```python
from build123d import *

# Parameters (mm, degrees)
ESQUISSE1_W             = 32.4
ESQUISSE1_H             = 21
BOSS_EXTRU_1_DEPTH      = 4
ESQUISSE2_W             = 4.7
ESQUISSE2_H             = 9.85
BOSS_EXTRU_2_DEPTH      = 12.3
ENL_V_MAT_EXTRU_1_REACH = 33.528
ESQUISSE3_R             = 0.95
CHANFREIN1_SIZE         = 1.915
CHANFREIN1_SIZE2        = 1.6
ESQUISSE4_R             = 1
ENL_V_MAT_EXTRU_2_DEPTH = 10
CONG_1_R                = 4.5
ESQUISSE5_R             = 1.5
ENL_V_MAT_EXTRU_3_DEPTH = 30.657924742
CHANFREIN2_SIZE         = 2.915
CHANFREIN2_SIZE2        = 2.24


with BuildPart() as part:
    # Esquisse1 → Boss.-Extru.1 (new body)
    with BuildSketch(Plane(origin=(0, 0, 0), x_dir=(1, 0, 0), z_dir=(0, 1, 0))):
        with Locations((0.75, -10.5)):
            Rectangle(ESQUISSE1_W, ESQUISSE1_H)
    extrude(amount=BOSS_EXTRU_1_DEPTH)

    # Esquisse2 → Boss.-Extru.2 (add)
    with BuildSketch(Plane(origin=(0, 4, 0), x_dir=(1, 0, 0), z_dir=(0, 1, 0))):
        Polygon((-15.45, 0), (-10.75, 0), (-10.75, -16.3), (16.95, -16.3), (16.95, -21), (-15.45, -21), align=None)
        with Locations((14.6, -4.925)):
            Rectangle(ESQUISSE2_W, ESQUISSE2_H)
    extrude(amount=BOSS_EXTRU_2_DEPTH)

    # Esquisse3 → Enlèv. mat.-Extru.1 (cut, up to next)
    with BuildSketch(Plane.XY.offset(21), mode=Mode.PRIVATE) as enl_v_mat_extru_1_sk1:
        with Locations((6.268372061, 10)):
            Circle(ESQUISSE3_R)
    enl_v_mat_extru_1_tool1 = extrude(enl_v_mat_extru_1_sk1.sketch, amount=-ENL_V_MAT_EXTRU_1_REACH, mode=Mode.PRIVATE) & part.part
    add(enl_v_mat_extru_1_tool1.solids().sort_by_distance((6.268372, 10, 21))[0], mode=Mode.SUBTRACT)

    # Chanfrein1
    chanfrein1_edges = [part.edges().sort_by_distance(p)[0] for p in [
        (5.318372061, 10, 16.3),
    ]]
    chanfrein1_side = [part.faces().sort_by_distance(p)[0] for p in [
        (3.073412496, 10.15125873, 16.3),
    ]]
    chamfer(chanfrein1_edges, length=CHANFREIN1_SIZE, length2=CHANFREIN1_SIZE2, reference=chanfrein1_side[0])

    # Esquisse4 → Enlèv. mat.-Extru.2 (cut)
    with BuildSketch(Plane(origin=(0, 0, 0), x_dir=(-1, 0, 0), z_dir=(0, 0, -1))):
        with Locations((-15.468268339, 10)):
            Circle(ESQUISSE4_R)
        with Locations((13.27835463, 10)):
            Circle(ESQUISSE4_R)
    extrude(amount=-ENL_V_MAT_EXTRU_2_DEPTH, mode=Mode.SUBTRACT)

    # Congé1
    cong_1_edges = [part.edges().sort_by_distance(p)[0] for p in [
        (14.6, 4, 9.85),
    ]]
    fillet(cong_1_edges, radius=CONG_1_R)

    # Esquisse5 → Enlèv. mat.-Extru.3 (cut, through all)
    with BuildSketch(Plane(origin=(0, 4, 0), x_dir=(1, 0, 0), z_dir=(0, 1, 0))):
        with Locations(Location((-6, -5, 0), (0, 0, 270))):
            Circle(ESQUISSE5_R)
        with Locations(Location((6, -5, 0), (0, 0, 270))):
            Circle(ESQUISSE5_R)
    extrude(amount=-ENL_V_MAT_EXTRU_3_DEPTH, mode=Mode.SUBTRACT)

    # Chanfrein2
    chanfrein2_edges = [part.edges().sort_by_distance(p)[0] for p in [
        (-6, 4, 3.5),
        (6, 4, 3.5),
    ]]
    chanfrein2_side = [part.faces().sort_by_distance(p)[0] for p in [
        (1.12179718, 4, 8.448141802),
    ]]
    chamfer(chanfrein2_edges, length=CHANFREIN2_SIZE, length2=CHANFREIN2_SIZE2, reference=chanfrein2_side[0])


solid = part.part
```
Input: part model. Units: mm. Frame: model coordinates. A direction names the side the tool comes from. Round coordinates to 2 decimals unless told otherwise and drop trailing zeros. Loops run counter-clockwise (first coordinate to the right, second up) from the corner with the lowest first, then second, coordinate; pieces in that order, holes last.
1) Section query D-D on y = 1. Return the cut outline in (x, z).
Ans:
outline: (-15.45, 0) - (16.95, 0) - (16.95, 21) - (-15.45, 21) - close; hole circle Ø3 at (-6, 5); hole circle Ø3 at (6, 5)
2) Material intervals for line 1 (X direction, y = 0.75, z = 5); line 2 (X direction, y = 8.5, z = 4); line 3 (X direction, y = 4.5, z = 14.75), sorted ascending.
Ans:
line 1: x = -15.45 to -7.5, -4.5 to 4.5, 7.5 to 16.95
line 2: x = -15.45 to -10.75, 12.25 to 16.95
line 3: x = -15.45 to -10.75
3) Set-up query: faces 1 (the flat face through (15, 12, 9.85)), 2 (the cylindrical face through (-12.541, 10.676, 4.93)), 3 (the conical face through (-7, 1.87, 3.7)), 4 (the flat face through (12.25, 10, 6)). Return all of +Z, -Z, +X, -X, +Y, -Y with unobstructed straight access to the full face (end or side cutting, diameter ignored); none if empty.
Ans:
face 1: +X, +Y
face 2: -Z
face 3: +Y
face 4: -Z, +Y
4) Section query C-C on y = 10. Return the cut outline in (x, z), plus the area to 3 significant figures.
Ans:
outline: (-15.45, 0) - (-14.28, 0) - (-14.28, 10) - (-12.28, 10) - (-12.28, 0) - (-10.75, 0) - (-10.75, 16.3) - (3.4, 16.3) - (5.32, 17.9) - (5.32, 21) - (-15.45, 21) - close; (7.22, 17.9) - (9.13, 16.3) - (16.95, 16.3) - (16.95, 21) - (7.22, 21) - close; (12.25, 0) - (14.47, 0) - (14.47, 9.85) - (12.25, 9.85) - close; (16.47, 0) - (16.95, 0) - (16.95, 9.85) - (16.47, 9.85) - close
area: 223 mm2
5) Pull-direction query (X, two-part tool) for faces 5 (the flat face through (1, 0, 10)), 6 (the flat face through (-15.45, 8, 11)), 7 (the flat face through (3, 4, 10)), 8 (the flat face through (16.95, 8, 8)); classes: released by +X, released by -X, zero draft, split by the parting line, or undercut.
Ans:
face 5: zero draft
face 6: released by -X
face 7: undercut
face 8: released by +X
6) Section query B-B on x = -6. Return the cut outline in (y, z) (3 decimals), plus the area to 3 significant figures.
Ans:
outline: (0, 0) - (4, 0) - (4, 0.585) - (1.76, 3.5) - (0, 3.5) - close; (0, 6.5) - (1.76, 6.5) - (4, 9.415) - (4, 16.3) - (16.3, 16.3) - (16.3, 21) - (0, 21) - close
area: 123 mm2
7) Pin query (flat end, axial travel): pin 1 (5 mm diameter, centred on x = 4.5, z = 14.5, fed in from -Y); pin 2 (3 mm diameter, centred on x = 1, z = 3, fed in from +Y); pin 3 (3.5 mm diameter, centred on x = -1.5, y = 11, fed in from -Z); pin 4 (4 mm diameter, centred on x = 6, z = 5, fed in from +Y). Return the tip coordinate at first contact, or that it passes through.
Ans:
pin 1: stops at y = 0
pin 2: stops at y = 4
pin 3: stops at z = 16.3
pin 4: stops at y = 2.14
8) Section query A-A on z = 5. Return the cut outline in (x, y) (3 decimals), plus the area to 3 significant figures.
Ans:
outline: (-15.45, 0) - (-7.5, 0) - (-7.5, 1.76) - (-10.415, 4) - (-10.75, 4) - (-10.75, 16.3) - (-15.45, 16.3) - close; (-4.5, 0) - (4.5, 0) - (4.5, 1.76) - (1.585, 4) - (-1.585, 4) - (-4.5, 1.76) - close; (7.5, 0) - (16.95, 0) - (16.95, 16.3) - (12.25, 16.3) - (12.25, 4) - (10.415, 4) - (7.5, 1.76) - close; hole circle Ø2 at (-13.278, 10); hole circle Ø2 at (15.468, 10)
area: 202 mm2
